The listing builds one solid part. Answer for the finished solid, in the listing's coordinates (mm). Face numbers are marked on the shaded views. A direction names the side the tool comes from. Give positions to 0.01 mm unless a question says otherwise; leave off trailing zeros. Loops run counter-clockwise (first coordinate to the right, second up) from the corner with the lowest first, then second, coordinate; pieces in that order, holes last. Notation, with made-up numbers: (75, 78.25) - (126, 78.25) arc R30 cw to (126, 103.25) - close; hole circle Ø8 at (85.5, -21.5). An arc over 180 degrees is marked (long way). Answer as CSV lines item,"result". Start each with the question number.
1) For a pull along Z with two mould halves and no side action, classify the marked faces 5, 6, 7 and 8 as pulls with the +Z half, pulls with the -Z half, needs draft (parallel to the pull), parting line crosses it, or undercut.
2) A cutting plane is placed at C-C (y = 9). Determine the outline of the cut face in (x, z), and give its area (4 significant figures).
3) Find the intervals of material crossed by line 1 along Z through (x, y) = (13.9, 17.3); line 2 along X through (y, z) = (8.75, 1); line 3 along Y through (x, z) = (0, -3.75), in increasing order.
4) A cutting plane is placed at B-B (z = -4.25). Determine the outline of the cut face in (x, y), and give its area (3 significant figures).
5) A cutting plane is placed at D-D (x = -8.5). Determine the outline of the cut face in (y, z), and give its area (3 significant figures).
6) A cutting plane is placed at A-A (x = 13.9). Determine the outline of the cut face in (y, z) (3 decimals), and give its area (3 significant figures).
7) Flat-ended cylindrical pins translate along their axes: pin 1 (3 mm diameter, centred on x = -3.5, z = 4.5, fed in from -Y); pin 2 (2.5 mm diameter, centred on x = -15, z = 1.5, fed in from +Y); pin 3 (1.9 mm diameter, centred on x = 13.9, z = 0, fed in from +Y); pin 4 (4 mm diameter, centred on y = 9.5, z = -0.5, fed in from -X). Find the tip coordinate at first contact, or state that the pin passes through.
8) For the marked faces 1, 2, 3 and 4, determine the directions among +Z, -Z, +X, -X, +Y, -Y from which every point of the face is accessible in a straight line to the end or side of a thin tool.
```python
from build123d import *

# Parameters (mm, degrees)
SKETCH1_W                      = 22.6
SKETCH1_H                      = 12.5
BOSS_EXTRUDE1_DEPTH            = 23
SKETCH2_W                      = 5
SKETCH2_H                      = 12.5
BOSS_EXTRUDE2_DEPTH            = 2.4
M2_CLEARANCE_HOLE1_D           = 2.4
M2_CLEARANCE_HOLE1_DEPTH       = 21.51
M2_CLEARANCE_HOLE1_CSINK_D     = 2.45
M2_CLEARANCE_HOLE1_CSINK_ANGLE = 90
M2_CLEARANCE_HOLE1_TIP         = 0.721032743
SKETCH5_R                      = 5.85
BOSS_EXTRUDE3_DEPTH            = 4.5


with BuildPart() as part:
    # Sketch1 → Boss-Extrude1 (new body)
    with BuildSketch(Plane(origin=(0, 0, 0), x_dir=(1, 0, 0), z_dir=(0, 1, 0))):
        Rectangle(SKETCH1_W, SKETCH1_H)
    extrude(amount=BOSS_EXTRUDE1_DEPTH)

    # Sketch2 → Boss-Extrude2 (add)
    with BuildSketch(Plane(origin=(0, 18.7, 0), x_dir=(1, 0, 0), z_dir=(0, 1, 0))):
        with Locations((13.8, 0)):
            Rectangle(SKETCH2_W, SKETCH2_H)
        with Locations((-13.8, 0)):
            Rectangle(SKETCH2_W, SKETCH2_H)
    extrude(amount=-BOSS_EXTRUDE2_DEPTH)

    # M2 Clearance Hole1
    with Locations(Plane(origin=(0, 18.7, 0), x_dir=(1, 0, 0), z_dir=(0, 1, 0))):
        with Locations((-13.9, 0), (13.9, 0)):
            CounterSinkHole(M2_CLEARANCE_HOLE1_D / 2, M2_CLEARANCE_HOLE1_CSINK_D / 2, depth=M2_CLEARANCE_HOLE1_DEPTH, counter_sink_angle=M2_CLEARANCE_HOLE1_CSINK_ANGLE)
            with Locations((0, 0, -(M2_CLEARANCE_HOLE1_DEPTH + M2_CLEARANCE_HOLE1_TIP / 2))):  # 118° drill point
                Cone(0, M2_CLEARANCE_HOLE1_D / 2, M2_CLEARANCE_HOLE1_TIP, mode=Mode.SUBTRACT)

    # Sketch5 → Boss-Extrude3 (add)
    with BuildSketch(Plane(origin=(0, 23, 0), x_dir=(1, 0, 0), z_dir=(0, 1, 0))):
        with Locations((-5.45, 0)):
            Circle(SKETCH5_R)
    extrude(amount=BOSS_EXTRUDE3_DEPTH)


solid = part.part
```
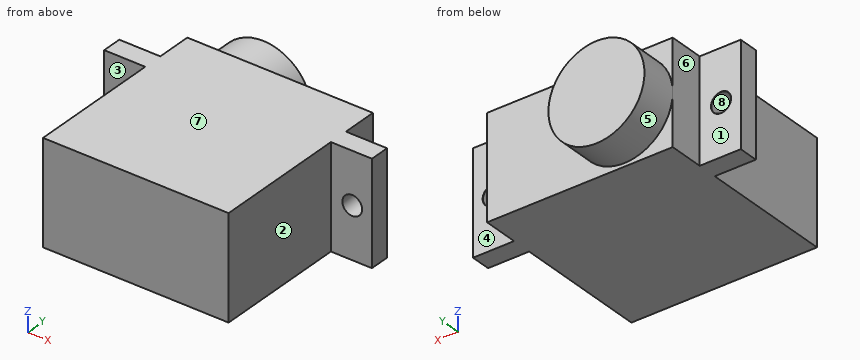
Ans:
1,face 5,"parting line crosses it"
1,face 6,"needs draft"
1,face 7,"pulls with the +Z half"
1,face 8,"undercut"
2,outline,"(-11.3, -6.25) - (11.3, -6.25) - (11.3, 6.25) - (-11.3, 6.25) - close"
2,area,"282.5 mm2"
3,line 1,"-6.25 to -1.2, 1.2 to 6.25"
3,line 2,"-11.3 to 11.3"
3,line 3,"0 to 23"
4,outline,"(-16.3, 16.3) - (-11.3, 16.3) - (-11.3, 0) - (11.3, 0) - (11.3, 16.3) - (16.3, 16.3) - (16.3, 18.7) - (11.3, 18.7) - (11.3, 23) - (-1.43, 23) - (-1.43, 27.5) - (-9.47, 27.5) - (-9.47, 23) - (-11.3, 23) - (-11.3, 18.7) - (-16.3, 18.7) - close"
4,area,"580 mm2"
5,outline,"(0, -6.25) - (23, -6.25) - (23, -4.99) - (27.5, -4.99) - (27.5, 4.99) - (23, 4.99) - (23, 6.25) - (0, 6.25) - close"
5,area,"332 mm2"
6,outline,"(16.3, -6.25) - (18.7, -6.25) - (18.7, -1.225) - (18.675, -1.2) - (16.3, -1.2) - close; (16.3, 1.2) - (18.675, 1.2) - (18.7, 1.225) - (18.7, 6.25) - (16.3, 6.25) - close"
6,area,"24.2 mm2"
7,pin 1,"y = 0"
7,pin 2,"y = 18.7"
7,pin 3,"through"
7,pin 4,"x = -11.3"
8,face 1,"+Z, -Z, -X, +Y"
8,face 2,"+Z, -Z, +X, -Y"
8,face 3,"+Z, -Z, -X, -Y"
8,face 4,"+Z, -Z, +X, +Y"
